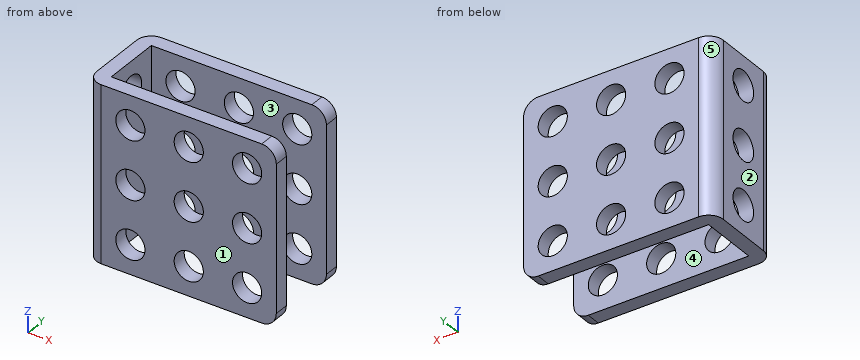
```python
from build123d import *

# Parameters (mm, degrees)
BOSS_EXTRUDE1_DEPTH  = 24
SKETCH2_R            = 2.05
CUT_EXTRUDE1_DEPTH   = 37
LPATTERN1_COUNT      = 3
LPATTERN1_PITCH      = 8
SKETCH3_R            = 2
CUT_EXTRUDE2_DEPTH   = 37.769552622
LPATTERN2_COUNT      = 3
LPATTERN2_PITCH      = 8
LPATTERN2_COUNT_DIR2 = 3
LPATTERN2_PITCH_DIR2 = 8
FILLET1_R            = 2


with BuildPart() as part:
    # Sketch1 → Boss-Extrude1 (new body)
    with BuildSketch(Plane.XY):
        Polygon((0, 0), (0, 10), (0, 12), (26, 12), (26, 10), (2, 10), (2, 2), (26, 2), (26, 0), align=None)
    extrude(amount=BOSS_EXTRUDE1_DEPTH)

    # Sketch2 → Cut-Extrude1 (cut, through all)
    with BuildSketch(Plane(origin=(2, 0, 0), x_dir=(0, 0, -1), z_dir=(1, 0, 0))):
        with Locations(Location((-20, 6, 0), (0, 0, 90))):
            Circle(SKETCH2_R)
    cut_extrude1 = extrude(amount=-CUT_EXTRUDE1_DEPTH, mode=Mode.SUBTRACT)

    # LPattern1: Cut-Extrude1 ×3
    with Locations(*[(0, 0, -i * LPATTERN1_PITCH) for i in range(1, LPATTERN1_COUNT)]):
        add(cut_extrude1, mode=Mode.SUBTRACT)

    # Sketch3 → Cut-Extrude2 (cut, symmetric)
    with BuildSketch(Plane(origin=(0, 2, 0), x_dir=(1, 0, 0), z_dir=(0, 1, 0))):
        with Locations(Location((22, -4, 0), (0, 0, 270))):
            Circle(SKETCH3_R)
    cut_extrude2 = extrude(amount=CUT_EXTRUDE2_DEPTH, both=True, mode=Mode.SUBTRACT)

    # LPattern2: Cut-Extrude2 3 × 3
    with Locations(*[(-j * LPATTERN2_PITCH_DIR2, 0, i * LPATTERN2_PITCH) for i in range(LPATTERN2_COUNT) for j in range(LPATTERN2_COUNT_DIR2) if (i, j) != (0, 0)]):
        add(cut_extrude2, mode=Mode.SUBTRACT)

    # Fillet1
    fillet1_edges = [part.edges().sort_by_distance(p)[0] for p in [
        (26, 1, 0),
        (0, 0, 12),
        (0, 12, 12),
        (26, 11, 24),
        (26, 1, 24),
        (26, 11, 0),
    ]]
    fillet(fillet1_edges, radius=FILLET1_R)


solid = part.part
```
Geometry: final body of the model. Coordinates: model frame, mm. Face numbers are marked on the shaded views. A direction names the side the tool comes from. Round coordinates to 2 decimals unless told otherwise and drop trailing zeros. Order: outer loops, then holes, each group sorted by start corner. A loop starts at its lowest first (then second) coordinate and runs counter-clockwise, first axis right, second up. Notation, with made-up numbers: (86, 36.25) - (142, 36.25) arc R23 ccw to (142, 54.25) - close; hole circle Ø5 at (2, 32.5). An arc over 180 degrees is marked (long way). Write item = value, one per line. Start each with the question number.
Q1. Pull-direction query (Y, two-part tool) for the marked faces 1, 2 and 3; classes: +Y half, -Y half, draft (parallel to the pull), parting line (faces both ways), or undercut.
Q2. Cut plane B-B on y = 6. Return the cut outline in (x, z), and give its area (3 significant figures).
Q3. Ray query, line 1 (Y direction, x = 24.5, z = 5.25); line 2 (Z direction, x = 0.55, y = 6); line 3 (Z direction, x = 5.5, y = 11.5). Return the intervals inside material, ascending. Write a range as from..to.
Q4. Cut plane D-D on z = 16.5. Return the cut outline in (x, y), and give its area (3 significant figures).
Q5. Access query for the marked faces 4 and 5. Directions: +Z, -Z, +X, -X, +Y, -Y. A direction counts if a zero-diameter tool reaches every point of the face in a straight line with its end or side. Return the directions, or none.
Q6. Cut plane A-A on x = 14. Give the number of separate pieces and of enclosed holes in the cut face, and give its area (3 significant figures).
Q7. Cut plane C-C on x = 19.5. Return the cut outline in (y, z), and give its area (3 significant figures).
Q8. Pin query (flat end, axial travel): pin 1 (1 mm diameter, centred on y = 5.5, z = 6, fed in from +X). Return the tip coordinate at first contact, or that it passes through.
Outcome:
q1.face_1 = -Y half
q1.face_2 = draft
q1.face_3 = undercut
q2.outline = (0, 0) - (2, 0) - (2, 1.95) - (0, 1.95) - close; (0, 6.05) - (2, 6.05) - (2, 9.95) - (0, 9.95) - close; (0, 14.05) - (2, 14.05) - (2, 17.95) - (0, 17.95) - close; (0, 22.05) - (2, 22.05) - (2, 24) - (0, 24) - close
q2.area = 23.4 mm^2
q3.line_1 = 0..2, 10..12
q3.line_2 = 0..1.95, 6.05..9.95, 14.05..17.95, 22.05..24
q3.line_3 = 0..2.06, 5.94..10.06, 13.94..18.06, 21.94..24
q4.outline = (0, 2) arc R2 ccw to (2, 0) - (26, 0) - (26, 2) - (2, 2) - (2, 10) - (26, 10) - (26, 12) - (2, 12) arc R2 ccw to (0, 10) - close
q4.area = 118 mm^2
q5.face_4 = +Z, -Z, +X
q5.face_5 = +Z, -Z, -X, +Y
q6.separate_pieces = 8
q6.enclosed_holes = 0
q6.area = 48.0 mm^2
q7.outline = (0, 0) - (2, 0) - (2, 24) - (0, 24) - close; (10, 0) - (12, 0) - (12, 24) - (10, 24) - close
q7.area = 96.0 mm^2
q8.pin_1 = 2
